Input: part model. Units: mm. Frame: model coordinates. A direction names the side the tool comes from. Give positions to 0.01 mm unless a question says otherwise; leave off trailing zeros. Loops run counter-clockwise (first coordinate to the right, second up) from the corner with the lowest first, then second, coordinate; pieces in that order, holes last. Notation, with made-up numbers: (19.5, -1) - (33.5, -1) arc R19 ccw to (33.5, 35) - close; hole circle Ø5 at (46, 89). An arc over 180 degrees is marked (long way). One line per item, written item: value.
from build123d import *

# Parameters (mm, degrees)
BOSS_EXTRUDE1_DEPTH = 1.27
BOSS_EXTRUDE2_START = 1.27
BOSS_EXTRUDE2_DEPTH = 1.27
BOSS_EXTRUDE3_DEPTH = 1.27
BOSS_EXTRUDE4_DEPTH = 2.794
BOSS_EXTRUDE5_DEPTH = 4.064
FILLET1_R           = 0.508
FILLET3_R           = 7.62


with BuildPart() as part:
    # Sketch1 → Boss-Extrude1 (new body)
    with BuildSketch(Plane.XY):
        with BuildLine():
            Line((0, 0), (42.291, 0))
            Line((42.291, 0), (42.291, 22.86))
            Line((42.291, 22.86), (23.0505, 22.86))
            Line((23.0505, 22.86), (23.0505, 3.81))
            ThreePointArc((23.0505, 3.81), (21.1455, 1.905), (19.2405, 3.81))
            Line((19.2405, 3.81), (19.2405, 22.86))
            Line((19.2405, 22.86), (0, 22.86))
            Line((0, 22.86), (0, 0))
        make_face()
    extrude(amount=BOSS_EXTRUDE1_DEPTH)

    # Sketch2 → Boss-Extrude2 (add)
    with BuildSketch(Plane(origin=(0, 0, 0), x_dir=(-1, 0, 0), z_dir=(0, 0, -1)).offset(BOSS_EXTRUDE2_START)):
        with BuildLine():
            Line((-23.0505, 22.86), (-39.8145, 22.86))
            Line((-39.8145, 22.86), (-39.8145, 0))
            Line((-39.8145, 0), (-23.0505, 0))
            Line((-23.0505, 0), (-19.2405, 0))
            Line((-19.2405, 0), (-2.4765, 0))
            Line((-2.4765, 0), (-2.4765, 22.86))
            Line((-2.4765, 22.86), (-19.2405, 22.86))
            Line((-19.2405, 22.86), (-19.2405, 3.81))
            ThreePointArc((-19.2405, 3.81), (-21.1455, 1.905), (-23.0505, 3.81))
            Line((-23.0505, 3.81), (-23.0505, 22.86))
        make_face()
    extrude(amount=-BOSS_EXTRUDE2_DEPTH)

    # Sketch3 → Boss-Extrude3 (add)
    with BuildSketch(Plane.XY.offset(1.27)):
        with BuildLine():
            Line((19.2405, 22.86), (2.4765, 22.86))
            Line((2.4765, 22.86), (2.4765, 0))
            Line((2.4765, 0), (19.2405, 0))
            Line((19.2405, 0), (23.0505, 0))
            Line((23.0505, 0), (39.8145, 0))
            Line((39.8145, 0), (39.8145, 22.86))
            Line((39.8145, 22.86), (23.0505, 22.86))
            Line((23.0505, 22.86), (23.0505, 3.81))
            ThreePointArc((23.0505, 3.81), (21.1455, 1.905), (19.2405, 3.81))
            Line((19.2405, 3.81), (19.2405, 22.86))
        make_face()
    extrude(amount=BOSS_EXTRUDE3_DEPTH)

    # Sketch5 → Boss-Extrude4 (add)
    with BuildSketch(Plane.XZ):
        with BuildLine():
            Line((-1.3335, -1.27), (43.6245, -1.27))
            Line((43.6245, -1.27), (38.1635, 13.97))
            ThreePointArc((38.1635, 13.97), (21.1455, 15.24), (4.1275, 13.97))
            Line((4.1275, 13.97), (-1.3335, -1.27))
        make_face()
    extrude(amount=BOSS_EXTRUDE4_DEPTH)

    # Sketch6 → Boss-Extrude5 (add)
    with BuildSketch(Plane.XZ.offset(2.794)):
        Polygon((1.761066667, 7.366), (13.9065, 7.366), (13.9065, -1.27), (-1.3335, -1.27), align=None)
        Polygon((28.3845, -1.27), (43.6245, -1.27), (40.529933333, 7.366), (28.3845, 7.366), align=None)
    extrude(amount=BOSS_EXTRUDE5_DEPTH)

    # Fillet1
    fillet1_edges = [part.edges().sort_by_distance(p)[0] for p in [
        (28.3845, -2.794, 3.048),
        (34.457216667, -2.794, 7.366),
        (13.9065, -2.794, 3.048),
        (7.833783333, -2.794, 7.366),
        (13.9065, -4.826, -1.27),
        (21.1455, -2.794, -1.27),
        (36.0045, -6.858, -1.27),
        (28.3845, -6.858, 3.048),
        (34.457216667, -6.858, 7.366),
        (42.077216667, -6.858, 3.048),
        (7.833783333, -6.858, 7.366),
        (13.9065, -6.858, 3.048),
        (6.2865, -6.858, -1.27),
        (0.213783333, -6.858, 3.048),
        (-1.3335, -3.429, -1.27),
        (28.3845, -4.826, -1.27),
        (43.6245, -3.429, -1.27),
        (38.1635, -1.397, 13.97),
        (4.1275, -1.397, 13.97),
    ]]
    fillet(fillet1_edges, radius=FILLET1_R)

    # Fillet3
    fillet3_edges = [part.edges().sort_by_distance(p)[0] for p in [
        (23.0505, 22.86, 0.635),
        (19.2405, 22.86, 0.635),
        (0, 22.86, 0.635),
        (42.291, 22.86, 0.635),
    ]]
    fillet(fillet3_edges, radius=FILLET3_R)


solid = part.part
Item 1: Section B-B, the plane x = 39. Output: boundary loops of the cut face in (y, z), and give its area (3 significant figures).
Verdict:
outline: (-6.86, -0.76) arc R0.51 ccw to (-6.35, -1.27) - (21.51, -1.27) - (21.51, 2.54) - (0, 2.54) - (0, 11.64) - (-2.79, 11.64) - (-2.79, 7.87) arc R0.51 cw to (-3.3, 7.37) - (-6.35, 7.37) arc R0.51 ccw to (-6.86, 6.86) - close
area: 153 mm^2
Item 2: Material intervals for L1, parallel to X at y = 11.75, z = 1.75; L2, parallel to Z at x = 19, y = 0.75; L3, parallel to Y at x = 12, z = 8.5, sorted ascending.
Verdict:
L1: x = 2.48 to 19.24, 23.05 to 39.81
L2: z = -1.27 to 2.54
L3: y = -2.79 to 0
Item 3: Section C-C, the plane y = -5. Output: boundary loops of the cut face in (x, z).
Verdict:
outline: (-1.09, -0.59) arc R0.51 ccw to (-0.61, -1.27) - (13.4, -1.27) arc R0.51 ccw to (13.91, -0.76) - (13.91, 7.37) - (1.76, 7.37) - close; (28.38, -0.76) arc R0.51 ccw to (28.89, -1.27) - (42.9, -1.27) arc R0.51 ccw to (43.38, -0.59) - (40.53, 7.37) - (28.38, 7.37) - close
Item 4: Section D-D, the plane x = 15. Output: boundary loops of the cut face in (y, z), and give its area (3 significant figures).
Verdict:
outline: (-2.79, -0.76) arc R0.51 ccw to (-2.29, -1.27) - (22.07, -1.27) - (22.07, 2.54) - (0, 2.54) - (0, 15.08) - (-2.79, 15.08) - close
area: 130 mm^2
Item 5: Pin query (flat end, axial travel): P1, Ø11.5, axis at x = 17.5, y = 10.5, coming from the +Z side; P2, Ø1.1, axis at y = 10, z = -0.5, coming from the +X side; P3, Ø4, axis at y = -3.5, z = 12.5, coming from the -X side. Return the tip coordinate at first contact, or that it passes through.
Verdict:
P1: stops at z = 2.54
P2: stops at x = 42.29
P3: stops at x = 2.93
Item 6: Draft query along X for faces 4 (the face through (35, -5, 7.366)), 5 (the face through (39.814, 11, -1)), 6 (the face through (21.187, 1.905, 0.608)). Return one class per face: pulls with the +X half, pulls with the -X half, needs draft (parallel to the pull), parting line crosses it, or undercut.
Verdict:
face 4: needs draft
face 5: pulls with the +X half
face 6: undercut
Item 7: Access query for faces 1 (the face through (8, -5, 7.366)), 2 (the face through (39.814, 10, 2)), 3 (the face through (28.384, -5, 3)). Directions: +Z, -Z, +X, -X, +Y, -Y. A direction counts if a zero-diameter tool reaches every point of the face in a straight line with its end or side. Return the directions, or none.
Verdict:
face 1: +Z, +X, -X, -Y
face 2: +Z, +X, +Y
face 3: +Z, -Z, -Y
Item 8: Section A-A, the plane y = 9. Output: boundary loops of the cut face in (x, z), and give its area (3 significant figures).
Verdict:
outline: (0, 0) - (2.48, 0) - (2.48, -1.27) - (19.24, -1.27) - (19.24, 2.54) - (2.48, 2.54) - (2.48, 1.27) - (0, 1.27) - close; (23.05, -1.27) - (39.81, -1.27) - (39.81, 0) - (42.29, 0) - (42.29, 1.27) - (39.81, 1.27) - (39.81, 2.54) - (23.05, 2.54) - close
area: 134 mm^2
